Check sheet for the modelled part. Datum: model origin and axes. Units: mm. Face numbers are marked on the shaded views. A direction names the side the tool comes from. Give positions to 0.01 mm unless a question says otherwise; leave off trailing zeros. Order: outer loops, then holes, each group sorted by start corner. A loop starts at its lowest first (then second) coordinate and runs counter-clockwise, first axis right, second up.
Autodesk Inventor part; units mm, degrees
ref_plane "YZ Plane" through (0, 0, 0) normal (1, 0, 0) x (0, 1, 0)
ref_plane "XZ Plane" through (0, 0, 0) normal (0, 1, 0) x (-1, 0, 0)
ref_plane "XY Plane" through (0, 0, 0) normal (0, 0, 1) x (1, 0, 0)
sketch "Sketch1" plane through (0, 0, 0) normal (0, 0, 1) x (1, 0, 0)
  line L0 (0, 38.2) -> (0, 0)
  line L1 (0, 0) -> (31, 0)
  line L2 (31, 0) -> (31, 4.8)
  line L3 (31, 4.8) -> (7.8, 4.8)
  line L4 (4.8, 7.8) -> (4.8, 38.2)
  line L5 (4.8, 38.2) -> (0, 38.2)
  arc A0 (4.8, 7.8) -> (7.8, 4.8) centre (7.8, 7.8) ccw
  dimension "d0" = 31
  dimension "d1" = 38.2
  dimension "d2" = 4.8
  dimension "d3" = 4.8
  dimension "d4" = 3
extrude "Extrusion1" add sketch "Sketch1" against normal blind 75
sketch "Sketch2" plane through (0, 0, 0) normal (-1, 0, 0) x (0, 0, 1)
  line L0 (0, 38.2) -> (-75, 38.2)
  line L1 (-75, 0) -> (-75, 38.2)
  point P0 (-69, 34.2)
  dimension "d7" = 4
  dimension "d8" = 6
hole "Hole1" at (0, 34.2, -69) direction (1, 0, 0) diameter 4.134 end through all
sketch "Sketch3" plane through (0, 0, 0) normal (-1, 0, 0) x (0, 0, 1)
  line L0 (0, 38.2) -> (-75, 38.2)
  line L1 (-75, 0) -> (-75, 38.2)
  line L2 (-35, 48.1735) -> (15.719, 48.1735)
  line L3 (15.719, 48.1735) -> (15.719, 22.2)
  line L4 (15.719, 22.2) -> (-35, 22.2)
  line L5 (-35, 22.2) -> (-35, 48.1735)
  dimension "d16" = 40
  dimension "d17" = 16
extrude "Extrusion2" cut sketch "Sketch3" against normal through all
sketch "Sketch4" plane through (0, 22.2, 0) normal (0, 1, 0) x (1, 0, 0)
  line L0 (4.8, 0) -> (0, 0)
  line L1 (0, 35) -> (4.8, 35)
  point P0 (2.4, 27)
  point P1 (2.4, 8)
  dimension "d20" = 8
  dimension "d21" = 8
hole "Hole2" at (2.4, 22.2, -27) at (2.4, 22.2, -8) direction (0, -1, 0) diameter 1.567 end through all
properties part number "Right Angle"
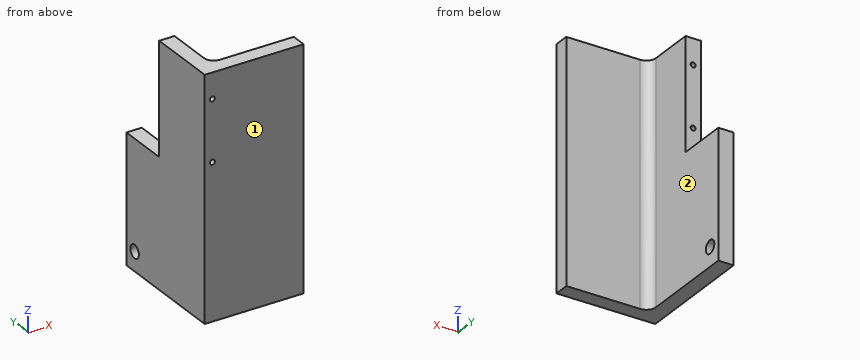
(1) Thickness scan on L1, parallel to Z at x = 2.4, y = 9.5; L2, parallel to X at y = 8.5, z = -8; L3, parallel to Z at x = 2, y = 16. Record the ranges inside material, lowest first.
(2) Sectioned sample at B-B (z = -8). Enter the section's corners in (x, y), plus the area to 3 significant figures.
(3) Go/stop test with flat-tipped pins: P1, Ø2.5, axis at x = 1.5, z = -22.5, coming from the +Y side; P2, Ø0.9, axis at x = 2.4, z = -27, coming from the -Y side; P3, Ø4, axis at x = 3.5, y = 32, coming from the +Z side; P4, Ø11.5, axis at x = 19, z = -41, coming from the +Y side. Record where each tip stops, or that it passes through.
(4) Sectioned sample at A-A (x = 2.4). Enter the section's corners in (y, z), plus the area to 3 significant figures.
(5) Tool access check on the marked faces 1 and 2. Record the directions out of +Z, -Z, +X, -X, +Y, -Y that give a thin tool (end or side, any length) a straight path to the whole face; none if there is none.
(6) Sectioned sample at D-D (z = -37). Enter the section's corners in (x, y), plus the area to 3 significant figures.
(7) Sectioned sample at C-C (y = 34.2). Enter the section's corners in (x, z).
Values follow:
1. L1: z = -75 to -27.78, -26.22 to -8.78, -7.22 to 0
1. L2: x = 0 to 1.62, 3.18 to 4.8
1. L3: z = -75 to -27.67, -26.33 to -8.67, -7.33 to 0
2. outline: (0, 0) - (1.62, 0) - (1.62, 22.2) - (0, 22.2) - close; (3.18, 0) - (31, 0) - (31, 4.8) - (7.8, 4.8) arc R3 cw to (4.8, 7.8) - (4.8, 22.2) - (3.18, 22.2) - close
2. area: 199 mm2
3. P1: stops at y = 22.2
3. P2: passes through
3. P3: stops at z = -35
3. P4: stops at y = 4.8
4. outline: (0, -75) - (38.2, -75) - (38.2, -35) - (22.2, -35) - (22.2, -27.78) - (0, -27.78) - close; (0, -26.22) - (22.2, -26.22) - (22.2, -8.78) - (0, -8.78) - close; (0, -7.22) - (22.2, -7.22) - (22.2, 0) - (0, 0) - close; hole circle Ø4.13 at (34.2, -69)
4. area: 2,220 mm2
5. face 1: +Z, -Z, +X, -X, -Y
5. face 2: +Z, -Z, +X, +Y
6. outline: (0, 0) - (31, 0) - (31, 4.8) - (7.8, 4.8) arc R3 cw to (4.8, 7.8) - (4.8, 38.2) - (0, 38.2) - close
6. area: 311 mm2
7. outline: (0, -75) - (4.8, -75) - (4.8, -71.07) - (0, -71.07) - close; (0, -66.93) - (4.8, -66.93) - (4.8, -35) - (0, -35) - close
